```python
from build123d import *

# Parameters (mm, degrees)
SKETCH_1_R          = 2
EXTRUDE_1_DEPTH     = 7
SKETCH_2_R          = 2.5
EXTRUDE_2_DEPTH     = 0.5
FILLET_1_R          = 0.5
SKETCH_3_R          = 1.5
CUT_EXTRUDE_1_DEPTH = 14


with BuildPart() as part:
    # 草图1 → 凸台-拉伸1 (new, symmetric)
    with BuildSketch(Plane.XY):
        Circle(SKETCH_1_R)
    extrude(amount=EXTRUDE_1_DEPTH, both=True)

    # 草图2 → 凸台-拉伸2 (add)
    with BuildSketch(Plane.XY.offset(7)):
        Circle(SKETCH_2_R)
    extrude(amount=EXTRUDE_2_DEPTH)

    # 圆角1
    fillet_1_edges = [part.edges().sort_by_distance(p)[0] for p in [
        (-2.5, 0, 7.5),
    ]]
    fillet(fillet_1_edges, radius=FILLET_1_R - 0.0001)  # a hair under: the kernel refuses the full size

    # 草图3 → 切除-拉伸1 (cut)
    with BuildSketch(Plane(origin=(0, 0, -7), x_dir=(-1, 0, 0), z_dir=(0, 0, -1))):
        Circle(SKETCH_3_R)
    extrude(amount=-CUT_EXTRUDE_1_DEPTH, mode=Mode.SUBTRACT)


solid = part.part
```
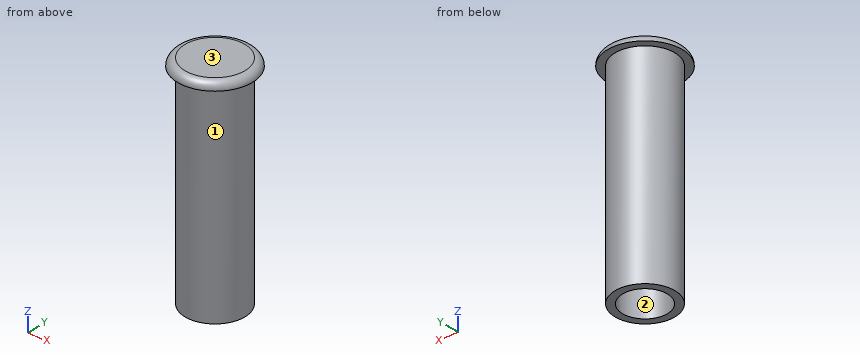
The model under review builds one solid part; all positions refer to its coordinate system, in mm. Face numbers are marked on the shaded views. Round coordinates to 2 decimals unless told otherwise and drop trailing zeros. Order: outer loops, then holes, each group sorted by start corner. A loop starts at its lowest first (then second) coordinate and runs counter-clockwise, first axis right, second up.
Item 1: Draft analysis for pull direction Y (two halves, no side actions). For the marked faces 1, 2 and 3, state which applies: released by +Y, released by -Y, zero draft, split by the parting line, or undercut.
Working result:
face 1: split by the parting line
face 2: undercut
face 3: zero draft
Item 2: For pin 1 (3 mm diameter, centred on x = 0.5, z = -4.5, fed in from +Y); pin 2 (3 mm diameter, centred on y = -1.5, z = 4.5, fed in from +X); pin 3 (1 mm diameter, centred on x = -1, z = 4.5, fed in from -Y), all flat-tipped, find the tip position at first contact; note any pin that passes through.
Working result:
pin 1: stops at y = 2
pin 2: stops at x = 2
pin 3: stops at y = -1.94
Item 3: Add section C-C, the plane z = 4.5. State the section outline as (x, y) points, and give its area (3 significant figures).
Working result:
outline: circle Ø4 at (0, 0); hole circle Ø3 at (0, 0)
area: 5.50 mm2
Item 4: To check wall thickness, follow probe 1 along Y at (x, z) = (0, 0.75); probe 2 along Z at (x, y) = (-0.25, 0.25); probe 3 along Y at (x, z) = (0.5, 1.5). State the ranges of each line that lie inside material, in increasing order.
Working result:
probe 1: y = -2 to -1.5, 1.5 to 2
probe 2: z = 7 to 7.5
probe 3: y = -1.94 to -1.41, 1.41 to 1.94
